```python
from build123d import *

# Parameters (mm, degrees)
SKETCH1_W           = 4
SKETCH1_H           = 4
BOSS_EXTRUDE1_DEPTH = 405


with BuildPart() as part:
    # Sketch1 → Boss-Extrude1 (new body)
    with BuildSketch(Plane(origin=(405, 0, 0), x_dir=(0, 0, -1), z_dir=(1, 0, 0))):
        with BuildLine():
            Line((-10.803382818, -20.752252101), (-6.5, -25.055634919))
            Line((-6.5, -25.055634919), (-6.5, -27.8))
            Line((-6.5, -27.8), (-10.9, -27.8))
            Line((-10.9, -27.8), (-10.9, -29.4))
            Line((-10.9, -29.4), (-10.3, -29.4))
            Line((-10.3, -29.4), (-10.3, -30))
            Line((-10.3, -30), (-1, -30))
            ThreePointArc((-1, -30), (-0.292893219, -29.707106781), (0, -29))
            Line((0, -29), (0, -19.7))
            Line((0, -19.7), (-0.6, -19.7))
            Line((-0.6, -19.7), (-0.6, -19.1))
            Line((-0.6, -19.1), (-2.2, -19.1))
            Line((-2.2, -19.1), (-2.2, -23.5))
            Line((-2.2, -23.5), (-4.944365081, -23.5))
            Line((-4.944365081, -23.5), (-9.247747899, -19.196617182))
            ThreePointArc((-9.247747899, -19.196617182), (-9.66365027, -18.400083987), (-9.549670182, -17.508765608))
            ThreePointArc((-9.549670182, -17.508765608), (-9, -15), (-9.549670182, -12.491234392))
            ThreePointArc((-9.549670182, -12.491234392), (-9.66365027, -11.599916013), (-9.247747899, -10.803382818))
            Line((-9.247747899, -10.803382818), (-4.944365081, -6.5))
            Line((-4.944365081, -6.5), (-2.2, -6.5))
            Line((-2.2, -6.5), (-2.2, -10.9))
            Line((-2.2, -10.9), (-0.6, -10.9))
            Line((-0.6, -10.9), (-0.6, -10.3))
            Line((-0.6, -10.3), (0, -10.3))
            Line((0, -10.3), (0, -1))
            ThreePointArc((0, -1), (-0.292893219, -0.292893219), (-1, 0))
            Line((-1, 0), (-10.3, 0))
            Line((-10.3, 0), (-10.3, -0.6))
            Line((-10.3, -0.6), (-10.9, -0.6))
            Line((-10.9, -0.6), (-10.9, -2.2))
            Line((-10.9, -2.2), (-6.5, -2.2))
            Line((-6.5, -2.2), (-6.5, -4.944365081))
            Line((-6.5, -4.944365081), (-10.803382818, -9.247747899))
            ThreePointArc((-10.803382818, -9.247747899), (-11.599916013, -9.66365027), (-12.491234392, -9.549670182))
            ThreePointArc((-12.491234392, -9.549670182), (-15, -9), (-17.508765608, -9.549670182))
            ThreePointArc((-17.508765608, -9.549670182), (-18.400083987, -9.66365027), (-19.196617182, -9.247747899))
            Line((-19.196617182, -9.247747899), (-23.5, -4.944365081))
            Line((-23.5, -4.944365081), (-23.5, -2.2))
            Line((-23.5, -2.2), (-19.1, -2.2))
            Line((-19.1, -2.2), (-19.1, -0.6))
            Line((-19.1, -0.6), (-19.7, -0.6))
            Line((-19.7, -0.6), (-19.7, 0))
            Line((-19.7, 0), (-40.3, 0))
            Line((-40.3, 0), (-40.3, -0.6))
            Line((-40.3, -0.6), (-40.9, -0.6))
            Line((-40.9, -0.6), (-40.9, -2.2))
            Line((-40.9, -2.2), (-36.5, -2.2))
            Line((-36.5, -2.2), (-36.5, -4.944365081))
            Line((-36.5, -4.944365081), (-40.803382818, -9.247747899))
            ThreePointArc((-40.803382818, -9.247747899), (-41.599916013, -9.66365027), (-42.491234392, -9.549670182))
            ThreePointArc((-42.491234392, -9.549670182), (-45, -9), (-47.508765608, -9.549670182))
            ThreePointArc((-47.508765608, -9.549670182), (-48.400083987, -9.66365027), (-49.196617182, -9.247747899))
            Line((-49.196617182, -9.247747899), (-53.5, -4.944365081))
            Line((-53.5, -4.944365081), (-53.5, -2.2))
            Line((-53.5, -2.2), (-49.1, -2.2))
            Line((-49.1, -2.2), (-49.1, -0.6))
            Line((-49.1, -0.6), (-49.7, -0.6))
            Line((-49.7, -0.6), (-49.7, 0))
            Line((-49.7, 0), (-59, 0))
            ThreePointArc((-59, 0), (-59.707106781, -0.292893219), (-60, -1))
            Line((-60, -1), (-60, -10.3))
            Line((-60, -10.3), (-59.4, -10.3))
            Line((-59.4, -10.3), (-59.4, -10.9))
            Line((-59.4, -10.9), (-57.8, -10.9))
            Line((-57.8, -10.9), (-57.8, -6.5))
            Line((-57.8, -6.5), (-55.055634919, -6.5))
            Line((-55.055634919, -6.5), (-50.752252101, -10.803382818))
            ThreePointArc((-50.752252101, -10.803382818), (-50.33634973, -11.599916013), (-50.450329818, -12.491234392))
            ThreePointArc((-50.450329818, -12.491234392), (-51, -15), (-50.450329818, -17.508765608))
            ThreePointArc((-50.450329818, -17.508765608), (-50.33634973, -18.400083987), (-50.752252101, -19.196617182))
            Line((-50.752252101, -19.196617182), (-55.055634919, -23.5))
            Line((-55.055634919, -23.5), (-57.8, -23.5))
            Line((-57.8, -23.5), (-57.8, -19.1))
            Line((-57.8, -19.1), (-59.4, -19.1))
            Line((-59.4, -19.1), (-59.4, -19.7))
            Line((-59.4, -19.7), (-60, -19.7))
            Line((-60, -19.7), (-60, -29))
            ThreePointArc((-60, -29), (-59.707106781, -29.707106781), (-59, -30))
            Line((-59, -30), (-49.7, -30))
            Line((-49.7, -30), (-49.7, -29.4))
            Line((-49.7, -29.4), (-49.1, -29.4))
            Line((-49.1, -29.4), (-49.1, -27.8))
            Line((-49.1, -27.8), (-53.5, -27.8))
            Line((-53.5, -27.8), (-53.5, -25.055634919))
            Line((-53.5, -25.055634919), (-49.196617182, -20.752252101))
            ThreePointArc((-49.196617182, -20.752252101), (-48.400083987, -20.33634973), (-47.508765608, -20.450329818))
            ThreePointArc((-47.508765608, -20.450329818), (-45, -21), (-42.491234392, -20.450329818))
            ThreePointArc((-42.491234392, -20.450329818), (-41.599916013, -20.33634973), (-40.803382818, -20.752252101))
            Line((-40.803382818, -20.752252101), (-36.5, -25.055634919))
            Line((-36.5, -25.055634919), (-36.5, -27.8))
            Line((-36.5, -27.8), (-40.9, -27.8))
            Line((-40.9, -27.8), (-40.9, -29.4))
            Line((-40.9, -29.4), (-40.3, -29.4))
            Line((-40.3, -29.4), (-40.3, -30))
            Line((-40.3, -30), (-19.7, -30))
            Line((-19.7, -30), (-19.7, -29.4))
            Line((-19.7, -29.4), (-19.1, -29.4))
            Line((-19.1, -29.4), (-19.1, -27.8))
            Line((-19.1, -27.8), (-23.5, -27.8))
            Line((-23.5, -27.8), (-23.5, -25.055634919))
            Line((-23.5, -25.055634919), (-19.196617182, -20.752252101))
            ThreePointArc((-19.196617182, -20.752252101), (-18.400083987, -20.33634973), (-17.508765608, -20.450329818))
            ThreePointArc((-17.508765608, -20.450329818), (-15, -21), (-12.491234392, -20.450329818))
            ThreePointArc((-12.491234392, -20.450329818), (-11.599916013, -20.33634973), (-10.803382818, -20.752252101))
        make_face()
        with Locations((-56.6, -26.6)):
            Rectangle(SKETCH1_W, SKETCH1_H, mode=Mode.SUBTRACT)
        with Locations((-56.6, -3.4)):
            Rectangle(SKETCH1_W, SKETCH1_H, mode=Mode.SUBTRACT)
        with Locations((-3.4, -26.6)):
            Rectangle(SKETCH1_W, SKETCH1_H, mode=Mode.SUBTRACT)
        with Locations((-3.4, -3.4)):
            Rectangle(SKETCH1_W, SKETCH1_H, mode=Mode.SUBTRACT)
        with BuildLine():
            Line((-39.247747899, -10.803382818), (-34.739339828, -6.294974747))
            ThreePointArc((-34.739339828, -6.294974747), (-34.414180701, -5.808339724), (-34.3, -5.234314575))
            Line((-34.3, -5.234314575), (-34.3, -2.2))
            Line((-34.3, -2.2), (-25.7, -2.2))
            Line((-25.7, -2.2), (-25.7, -5.234314575))
            ThreePointArc((-25.7, -5.234314575), (-25.585819299, -5.808339724), (-25.260660172, -6.294974747))
            Line((-25.260660172, -6.294974747), (-20.752252101, -10.803382818))
            ThreePointArc((-20.752252101, -10.803382818), (-20.33634973, -11.599916013), (-20.450329818, -12.491234392))
            ThreePointArc((-20.450329818, -12.491234392), (-21, -15), (-20.450329818, -17.508765608))
            ThreePointArc((-20.450329818, -17.508765608), (-20.33634973, -18.400083987), (-20.752252101, -19.196617182))
            Line((-20.752252101, -19.196617182), (-25.260660172, -23.705025253))
            ThreePointArc((-25.260660172, -23.705025253), (-25.585819299, -24.191660276), (-25.7, -24.765685425))
            Line((-25.7, -24.765685425), (-25.7, -27.8))
            Line((-25.7, -27.8), (-34.3, -27.8))
            Line((-34.3, -27.8), (-34.3, -24.765685425))
            ThreePointArc((-34.3, -24.765685425), (-34.414180701, -24.191660276), (-34.739339828, -23.705025253))
            Line((-34.739339828, -23.705025253), (-39.247747899, -19.196617182))
            ThreePointArc((-39.247747899, -19.196617182), (-39.66365027, -18.400083987), (-39.549670182, -17.508765608))
            ThreePointArc((-39.549670182, -17.508765608), (-39, -15), (-39.549670182, -12.491234392))
            ThreePointArc((-39.549670182, -12.491234392), (-39.66365027, -11.599916013), (-39.247747899, -10.803382818))
        make_face(mode=Mode.SUBTRACT)
        with BuildLine():
            ThreePointArc((-47.802270236, -17.096969605), (-48.5, -15), (-47.802270236, -12.903030395))
            ThreePointArc((-47.802270236, -12.903030395), (-47.828427125, -12.171572875), (-47.096969605, -12.197729764))
            ThreePointArc((-47.096969605, -12.197729764), (-45, -11.5), (-42.903030395, -12.197729764))
            ThreePointArc((-42.903030395, -12.197729764), (-42.171572875, -12.171572875), (-42.197729764, -12.903030395))
            ThreePointArc((-42.197729764, -12.903030395), (-41.5, -15), (-42.197729764, -17.096969605))
            ThreePointArc((-42.197729764, -17.096969605), (-42.171572875, -17.828427125), (-42.903030395, -17.802270236))
            ThreePointArc((-42.903030395, -17.802270236), (-45, -18.5), (-47.096969605, -17.802270236))
            ThreePointArc((-47.096969605, -17.802270236), (-47.828427125, -17.828427125), (-47.802270236, -17.096969605))
        make_face(mode=Mode.SUBTRACT)
        with BuildLine():
            ThreePointArc((-12.197729764, -12.903030395), (-11.5, -15), (-12.197729764, -17.096969605))
            ThreePointArc((-12.197729764, -17.096969605), (-12.171572875, -17.828427125), (-12.903030395, -17.802270236))
            ThreePointArc((-12.903030395, -17.802270236), (-15, -18.5), (-17.096969605, -17.802270236))
            ThreePointArc((-17.096969605, -17.802270236), (-17.828427125, -17.828427125), (-17.802270236, -17.096969605))
            ThreePointArc((-17.802270236, -17.096969605), (-18.5, -15), (-17.802270236, -12.903030395))
            ThreePointArc((-17.802270236, -12.903030395), (-17.828427125, -12.171572875), (-17.096969605, -12.197729764))
            ThreePointArc((-17.096969605, -12.197729764), (-15, -11.5), (-12.903030395, -12.197729764))
            ThreePointArc((-12.903030395, -12.197729764), (-12.171572875, -12.171572875), (-12.197729764, -12.903030395))
        make_face(mode=Mode.SUBTRACT)
    extrude(amount=-BOSS_EXTRUDE1_DEPTH)


solid = part.part
```
The model under review builds one solid part; all positions refer to its coordinate system, in mm. A direction names the side the tool comes from. Give positions to 0.01 mm unless a question says otherwise; leave off trailing zeros.
(1) Consider section A-A, the plane x = 230. Give the number of separate pieces and of enclosed holes in the cut face, and give its area (3 significant figures).
(2) Tool access review of faces 4 (the flat face through (205, -2.2, 30)), 5 (the flat face through (205, 0, 6)): name each direction out of +Z, -Z, +X, -X, +Y, -Y from which nothing blocks a thin tool from reaching the whole face with its end or side.
(3) For P1, Ø0.7, axis at x = 161, y = -29.5, coming from the -Z side; P2, Ø2, axis at x = 108, z = 9.5, coming from the +Y side; P3, Ø1, axis at x = 129.5, z = 13.5, coming from the -Y side, all flat-tipped, find the tip position at first contact; note any pin that passes through.
(4) The part is to be moulded in two halves that separate along Y. For faces 1 (the flat face through (205, -30, 54)), 2 (the flat face through (205, -24, 60)), 3 (the flat face through (205, -27.8, 30)), say which applies: released by +Y, released by -Y, zero draft, split by the parting line, or undercut.
(5) To check wall thickness, follow L1, parallel to Z at x = 274.5, y = -3; L2, parallel to Z at x = 120.5, y = -22; L3, parallel to Y at x = 23, z = 57.5. State the ranges of each line that lie inside material, in increasing order.
Returned:
1. separate pieces: 1
1. enclosed holes: 7
1. area: 576 mm2
2. face 4: +X, -X
2. face 5: +Z, -Z, +X, -X, +Y
3. P1: stops at z = 0.01
3. P2: stops at y = 0
3. P3: stops at y = -20.92
4. face 1: released by -Y
4. face 2: zero draft
4. face 3: undercut
5. L1: z = 0 to 1.4, 5.4 to 6.5, 23.5 to 25.7, 34.3 to 36.5, 53.5 to 54.6, 58.6 to 60
5. L2: z = 0 to 2.2, 6.44 to 9.56, 20.44 to 23.56, 36.44 to 39.56, 50.44 to 53.56, 57.8 to 60
5. L3: y = -30 to -28.6, -24.6 to -23.5, -6.5 to -5.4, -1.4 to 0
